Could you check a few things on this drawing? It's one solid part, dimensions in mm from its lowest x, y, z. A direction names the side the tool comes from. Coordinates: 2 decimals unless noted, no trailing zeros. Loops run counter-clockwise (first coordinate to the right, second up) from the corner with the lowest first, then second, coordinate; pieces in that order, holes last. Notation, with made-up numbers: (-32, -8) -> (-8, -8) arc R22 cw to (-8, -1) -> close; hole circle Ø9 at (-34, 46). An arc over 180 degrees is marked (long way). One line per question, with ' | ' between items. Start each with the question number.
(1) Suppose I cut it at C-C (x = 28). Please give me the cut outline in (y, z), plus the area to 3 significant figures.
(2) If I drill on line 1 along X through (y, z) = (46, 20); line 2 along Z through (x, y) = (1, 56); line 3 along Z through (x, y) = (11.5, 9.5), over which ranges is the centre line in solid material (lowest first)?
(3) I'm going to push flat-ended pins straight in: pin 1 Ø1.5 at (x, z) = (6.5, 19) entering from -Y; pin 2 Ø5 at (x, z) = (27, 9) entering from +Y; pin 3 Ø4 at (x, y) = (22.5, 17) entering from +Z; pin 4 Ø2.5 at (y, z) = (56, 18) entering from -X. Where does each tip first touch, or does it pass through?
(4) Suppose I cut it at B-B (z = 14). Please give me the cut outline in (x, y), plus the area to 3 significant figures.
(5) If we mould it in two halves opening along X, with no side actions, what happens to the marked faces 3, 4 and 5? For each: pulls with the +X half, pulls with the -X half, needs draft (parallel to the pull), parting line crosses it, or undercut.
(6) Suppose I cut it at D-D (z = 18). Please give me the cut outline in (x, y).
(7) Which directions (+Z, -Z, +X, -X, +Y, -Y) give clear straight access to the entire face, cutting with the end or side of a thin tool? Please do the marked faces 1 and 2.
(8) Suppose I cut it at A-A (y = 27). Please give me the cut outline in (x, z), plus the area to 3 significant figures.
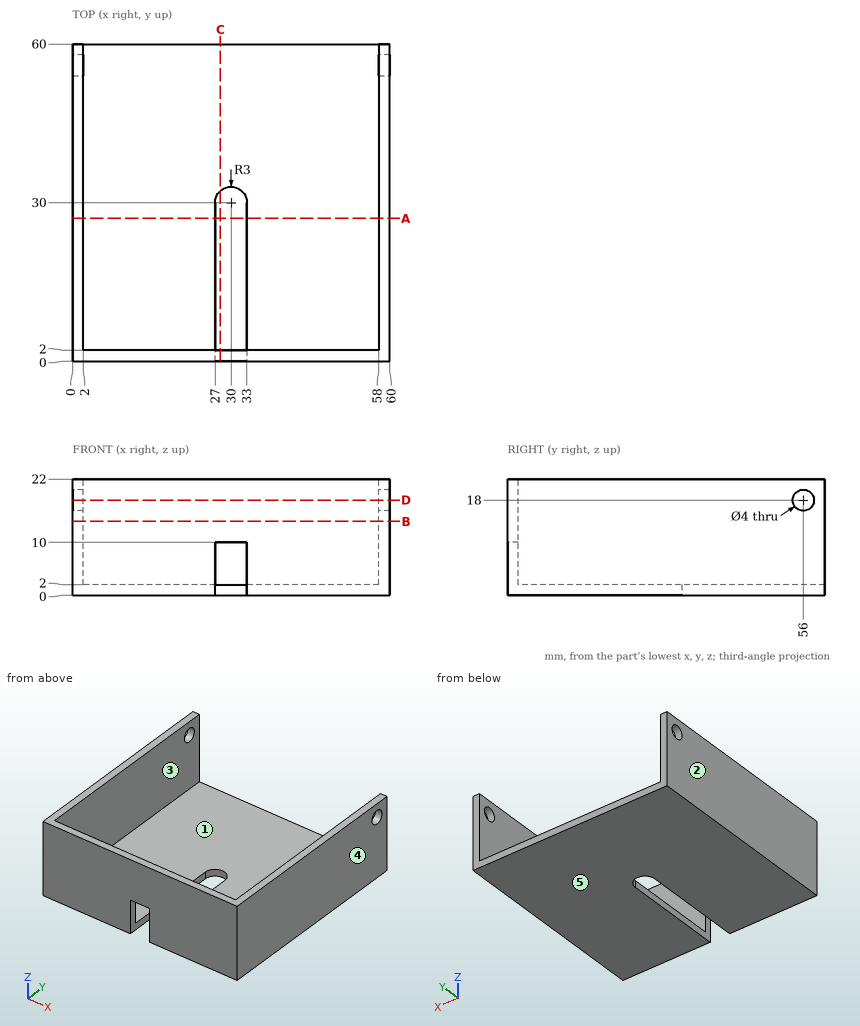
Checks:
1) outline: (0, 10) -> (2, 10) -> (2, 22) -> (0, 22) -> close; (32.24, 0) -> (60, 0) -> (60, 2) -> (32.24, 2) -> close | area: 79.5 mm^2
2) line 1: x = 0 to 2, 58 to 60 | line 2: z = 0 to 16, 20 to 22 | line 3: z = 0 to 2
3) pin 1: stops at y = 0 | pin 2: stops at y = 2 | pin 3: stops at z = 2 | pin 4: passes through
4) outline: (0, 0) -> (60, 0) -> (60, 60) -> (58, 60) -> (58, 2) -> (2, 2) -> (2, 60) -> (0, 60) -> close | area: 352 mm^2
5) face 3: undercut | face 4: pulls with the +X half | face 5: needs draft
6) outline: (0, 0) -> (60, 0) -> (60, 54) -> (58, 54) -> (58, 2) -> (2, 2) -> (2, 54) -> (0, 54) -> close; (0, 58) -> (2, 58) -> (2, 60) -> (0, 60) -> close; (58, 58) -> (60, 58) -> (60, 60) -> (58, 60) -> close
7) face 1: +Z, +Y | face 2: +Z, -Z, -X, +Y, -Y
8) outline: (0, 0) -> (27, 0) -> (27, 2) -> (2, 2) -> (2, 22) -> (0, 22) -> close; (33, 0) -> (60, 0) -> (60, 22) -> (58, 22) -> (58, 2) -> (33, 2) -> close | area: 188 mm^2
